Could you check a few things on this model? Use its own coordinates, in mm. Face numbers are marked on the shaded views. A direction names the side the tool comes from. Coordinates: 2 decimals unless noted, no trailing zeros. Order: outer loops, then holes, each group sorted by start corner. A loop starts at its lowest first (then second) coordinate and runs counter-clockwise, first axis right, second up. Notation, with made-up numbers: (20.5, 88) - (36.5, 88) arc R13 cw to (36.5, 104) - close; hole circle Ø9 at (-4.5, 50.25). An arc over 180 degrees is marked (long way). Answer as CSV lines item,"result". Start each with the question number.
1. I want a section at C-C, the plane z = 5. List the corners of the cut face in (x, y) for me, and give its area (3 significant figures).
2. I need wall thicknesses on probe 1 along Z at (x, y) = (13.5, -7); probe 2 along Z at (x, y) = (-28, 3); probe 3 along X at (y, z) = (9.5, 30). Which ranges of each line are inside material? Lowest first, please.
3. For pin 1 (7 mm diameter, centred on y = -3, z = 31, fed in from +X); pin 2 (7.5 mm diameter, centred on x = 17, y = -0.5, fed in from +Z); pin 3 (5.5 mm diameter, centred on x = -28.5, y = -3, fed in from +Z), each with a flat end and sliding along its axis, tell me the tip position at first contact or that it passes through.
4. For the marked faces 1, 2 and 3, which set-ups out of +Z, -Z, +X, -X, +Y, -Y let a thin tool reach every point of the face, with its end or its side?
5. I want a section at B-B, the plane x = -12.5. List the corners of the cut face in (y, z) for me, and give its area (3 significant figures).
6. I want a section at A-A, the plane y = 5.25. List the corners of the cut face in (x, z) for me, and give its area (3 significant figures).
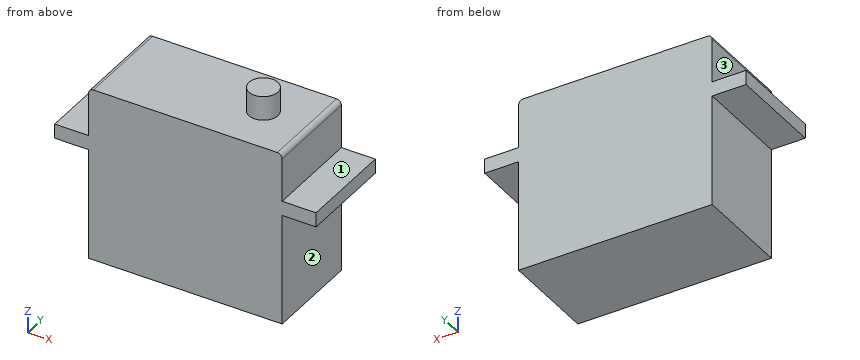
from build123d import *

# Parameters (mm, degrees)
ESQUISSE1_W        = 40
ESQUISSE1_H        = 20
BOSS_EXTRU_1_DEPTH = 36
ESQUISSE2_W        = 3
ESQUISSE2_H        = 20
BOSS_EXTRU_2_DEPTH = 7
ESQUISSE3_W        = 3
ESQUISSE3_H        = 20
BOSS_EXTRU_3_DEPTH = 7
ESQUISSE4_R        = 3
BOSS_EXTRU_4_DEPTH = 5
CONG_1_R           = 1


with BuildPart() as part:
    # Esquisse1 → Boss.-Extru.1 (new body)
    with BuildSketch(Plane.XY):
        with Locations((-4.886048962, 0.290697674)):
            Rectangle(ESQUISSE1_W, ESQUISSE1_H)
    extrude(amount=BOSS_EXTRU_1_DEPTH)

    # Esquisse2 → Boss.-Extru.2 (add)
    with BuildSketch(Plane(origin=(15.113951038, 0, 0), x_dir=(0, 0, -1), z_dir=(1, 0, 0))):
        with Locations((-24.5, 0.290697674)):
            Rectangle(ESQUISSE2_W, ESQUISSE2_H)
    extrude(amount=BOSS_EXTRU_2_DEPTH)

    # Esquisse3 → Boss.-Extru.3 (add)
    with BuildSketch(Plane.ZY.offset(24.886048962)):
        with Locations((24.5, 0.290697674)):
            Rectangle(ESQUISSE3_W, ESQUISSE3_H)
    extrude(amount=BOSS_EXTRU_3_DEPTH)

    # Esquisse4 → Boss.-Extru.4 (add)
    with BuildSketch(Plane.XY.offset(36)):
        with Locations((5.113951038, 0.290697674)):
            Circle(ESQUISSE4_R)
    extrude(amount=BOSS_EXTRU_4_DEPTH)

    # Congé1
    cong_1_edges = [part.edges().sort_by_distance(p)[0] for p in [
        (15.113951038, 0.290697674, 36),
        (-24.886048962, 0.290697674, 36),
    ]]
    fillet(cong_1_edges, radius=CONG_1_R)


solid = part.part
Solved:
1,outline,"(-24.89, -9.71) - (15.11, -9.71) - (15.11, 10.29) - (-24.89, 10.29) - close"
1,area,"800 mm2"
2,probe 1,"z = 0 to 36"
2,probe 2,"z = 23 to 26"
2,probe 3,"x = -24.89 to 15.11"
3,pin 1,"stops at x = 15.11"
3,pin 2,"stops at z = 36"
3,pin 3,"stops at z = 26"
4,face 1,"+Z, +X, +Y, -Y"
4,face 2,"-Z, +X, +Y, -Y"
4,face 3,"+Z, -X, +Y, -Y"
5,outline,"(-9.71, 0) - (10.29, 0) - (10.29, 36) - (-9.71, 36) - close"
5,area,"720 mm2"
6,outline,"(-31.89, 23) - (-24.89, 23) - (-24.89, 0) - (15.11, 0) - (15.11, 23) - (22.11, 23) - (22.11, 26) - (15.11, 26) - (15.11, 35) arc R1 ccw to (14.11, 36) - (-23.89, 36) arc R1 ccw to (-24.89, 35) - (-24.89, 26) - (-31.89, 26) - close"
6,area,"1,480 mm2"
